Can you work these out from the model? Positions are in its coordinate system, mm. A direction names the side the tool comes from. Give positions to 0.01 mm unless a question says otherwise; leave off trailing zeros. Order: outer loops, then holes, each group sorted by start corner. A loop starts at its lowest first (then second) coordinate and runs counter-clockwise, first axis right, second up. Notation, with made-up numbers: M 34.25,51 L 40.25,51 A25 ccw 40.25,67 Z; hole C 8.25,-27 d4. An arc over 180 degrees is marked long. One line per question, with ' | ' between items. Start each with the question number.
1) Thinking about a two-plate mould opening in X: for faces 1 (the flat face through (-18, 17, -12)), 2 (the flat face through (0, 18, -2.5)), 3 (the cylindrical face through (0, 10, -10)), which applies, +X half, -X half, draft (parallel to the pull), parting line (faces both ways), or undercut?
2) Please list where these lines run through material, in increasing order: line 1 along X through (y, z) = (-15, -2.5); line 2 along Y through (x, z) = (-6, -13.25); line 3 along Y through (x, z) = (-11, -13.5). Write a range as [from, to].
3) I'm going to push flat-ended pins straight in: pin 1 Ø4 at (x, z) = (-5.5, -5) entering from -Y; pin 2 Ø2 at (x, z) = (-5.5, -3) entering from -Y; pin 3 Ø6 at (x, y) = (8, -17.5) entering from +Z; pin 4 Ø12 at (y, z) = (22, -7) entering from +X. Where does each tip first touch, or does it pass through?
4) If we section it at C-C, the plane y = -11: Please give me the cut outline in (x, z), plus the area to 3 significant figures.
5) For faces 4 (the flat face through (-15, -9, -10)), 5 (the flat face through (-10.2, 0.7, 0)), 6 (the flat face through (-5, -18, -8)), which set-ups out of +Z, -Z, +X, -X, +Y, -Y let a thin tool reach every point of the face, with its end or its side?
6) If we section it at A-A, the plane y = -5: Please give me the cut outline in (x, z), plus the area to 3 significant figures.
7) If we section it at B-B, the plane z = -10.5: Please give me the cut outline in (x, y).
8) If we section it at D-D, the plane z = -7: Please give me the cut outline in (x, y), plus the area to 3 significant figures.
```python
from build123d import *
from build123d.topology import SkipClean

# Parameters (mm, degrees)
BIG_CYL_DEPTH       = 20
HALF_CIRCLE_DEPTH   = 10
SMALL_CYL_DEPTH     = 10
HALF_START          = -10
HALF_CIRCLE_2_DEPTH = 10
SMAL_START          = -10
SMAL_CYL_2_DEPTH    = 10
LONG_CYL_DEPTH      = 18
BASE_DEPTH          = 10


with BuildPart() as part:
    # Sketch1 → big cyl (new body)
    with BuildSketch(Plane.XY):
        with BuildLine():
            Line((-15, 0), (-15, -14))
            Line((-15, -14), (-5, -14))
            Line((-5, -14), (-5, -8.660254038))
            ThreePointArc((-5, -8.660254038), (0, 10), (5, -8.660254038))
            Line((5, -8.660254038), (5, -14))
            Line((5, -14), (15, -14))
            Line((15, -14), (15, 0))
            ThreePointArc((15, 0), (0, 15), (-15, 0))
        make_face()
    extrude(amount=-BIG_CYL_DEPTH)

    # Sketch2 → half circle (add)
    with BuildSketch(Plane.ZY.offset(15)):
        with BuildLine():
            Line((-14, -14), (-20, -14))
            ThreePointArc((-20, -14), (-10, -24), (0, -14))
            Line((0, -14), (-6, -14))
            ThreePointArc((-6, -14), (-10, -18), (-14, -14))
        make_face()
    extrude(amount=-HALF_CIRCLE_DEPTH)

    # Sketch2_5 → small cyl (cut)
    with SkipClean():  # the faces are left unmerged after this step: merging them gives an invalid solid
        with BuildSketch(Plane.ZY.offset(15)):
            with BuildLine():
                Line((-14, -14), (-6, -14))
                ThreePointArc((-6, -14), (-10, -10), (-14, -14))
            make_face()
        extrude(amount=-SMALL_CYL_DEPTH, mode=Mode.SUBTRACT)

    # Sketch4 → half circle 2 (add)
    with SkipClean():  # the faces are left unmerged after this step: merging them gives an invalid solid
        with BuildSketch(Plane(origin=(15, 0, 0), x_dir=(0, 0, -1), z_dir=(1, 0, 0)).offset(HALF_START)):
            with BuildLine():
                Line((6, -14), (0, -14))
                ThreePointArc((0, -14), (10, -24), (20, -14))
                Line((20, -14), (14, -14))
                ThreePointArc((14, -14), (10, -18), (6, -14))
            make_face()
        extrude(amount=HALF_CIRCLE_2_DEPTH)

    # Sketch4_4 → smal cyl 2 (cut)
    with SkipClean():  # the faces are left unmerged after this step: merging them gives an invalid solid
        with BuildSketch(Plane(origin=(15, 0, 0), x_dir=(0, 0, -1), z_dir=(1, 0, 0)).offset(SMAL_START)):
            with BuildLine():
                ThreePointArc((14, -14), (10, -10), (6, -14))
                Line((6, -14), (14, -14))
            make_face()
            with BuildLine():
                Line((14, -14), (6, -14))
                ThreePointArc((6, -14), (10, -18), (14, -14))
            make_face()
        extrude(amount=SMAL_CYL_2_DEPTH, mode=Mode.SUBTRACT)

    # Sketch5 → long cyl (add, symmetric)
    with SkipClean():  # the faces are left unmerged after this step: merging them gives an invalid solid
        with BuildSketch(Plane(origin=(0, 0, 0), x_dir=(0, 0, -1), z_dir=(1, 0, 0))):
            with BuildLine():
                ThreePointArc((8, 29.228416147), (4.031331807, 26.541475531), (2.5, 22))
                ThreePointArc((2.5, 22), (10, 14.5), (17.5, 22))
                ThreePointArc((17.5, 22), (15.968668193, 26.541475531), (12, 29.228416147))
                Line((12, 29.228416147), (12, 26.582575695))
                ThreePointArc((12, 26.582575695), (14.183300133, 24.738612788), (15, 22))
                ThreePointArc((15, 22), (7.261387212, 17.816699867), (8, 26.582575695))
                Line((8, 26.582575695), (8, 29.228416147))
            make_face()
        extrude(amount=LONG_CYL_DEPTH, both=True)

    # Sketch5_3 → base (add, symmetric)
    with SkipClean():  # the faces are left unmerged after this step: merging them gives an invalid solid
        with BuildSketch(Plane(origin=(0, 0, 0), x_dir=(0, 0, -1), z_dir=(1, 0, 0))):
            with BuildLine():
                ThreePointArc((17.5, 22), (10, 14.5), (2.5, 22))
                Line((2.5, 22), (2.5, 10.5))
                Line((2.5, 10.5), (17.5, 10.5))
                Line((17.5, 10.5), (17.5, 22))
            make_face()
        extrude(amount=BASE_DEPTH, both=True)


solid = part.part
```
Results found:
1) face 1: -X half | face 2: draft | face 3: undercut
2) line 1: x = [-15, -5], [5, 15] | line 2: y = [-23.46, -16.33], [-11.67, -8], [8, 18.2], [25.8, 28.76] | line 3: y = [-23.37, -15.94], [-12.06, 10.2], [15.37, 18.43], [25.57, 28.63]
3) pin 1: stops at y = -23.54 | pin 2: stops at y = -22 | pin 3: stops at z = -0.01 | pin 4: stops at x = 18
4) outline: M -15,-20 L -5,-20 L -5,-12.65 L -15,-12.65 Z; M -15,-7.35 L -5,-7.35 L -5,0 L -15,0 Z; M 5,-20 L 15,-20 L 15,-12.65 L 5,-12.65 Z; M 5,-7.35 L 15,-7.35 L 15,0 L 5,0 Z | area: 294 mm²
5) face 4: +Z, -Z, -X, -Y | face 5: +Z, +X, -X, +Y, -Y | face 6: +Z, -Z, -Y
6) outline: M -15,-20 L -8.66,-20 L -8.66,0 L -15,0 Z; M 8.66,-20 L 15,-20 L 15,0 L 8.66,0 Z | area: 254 mm²
7) outline: M -18,14.52 L -10,14.52 L -10,11.18 A15 ccw -15,0 L -15,-10.03 L -5,-10.03 L -5,-8.66 A10 cw long 5,-8.66 L 5,-10.03 L 15,-10.03 L 15,0 A15 ccw 10,11.18 L 10,14.52 L 18,14.52 L 18,17.03 L -18,17.03 Z; M -15,-23.99 L -5,-23.99 L -5,-17.97 L -15,-17.97 Z; M 5,-23.99 L 15,-23.99 L 15,-17.97 L 5,-17.97 Z
8) outline: M -18,15.13 L -10,15.13 L -10,11.18 A15 ccw -15,0 L -15,-11.35 L -5,-11.35 L -5,-8.66 A10 cw long 5,-8.66 L 5,-11.35 L 15,-11.35 L 15,0 A15 ccw 10,11.18 L 10,15.13 L 18,15.13 L 18,18 L -18,18 Z; M -18,26 L 18,26 L 18,28.87 L -18,28.87 Z; M -15,-23.54 L -5,-23.54 L -5,-16.65 L -15,-16.65 Z; M 5,-23.54 L 15,-23.54 L 15,-16.65 L 5,-16.65 Z | area: 733 mm²
